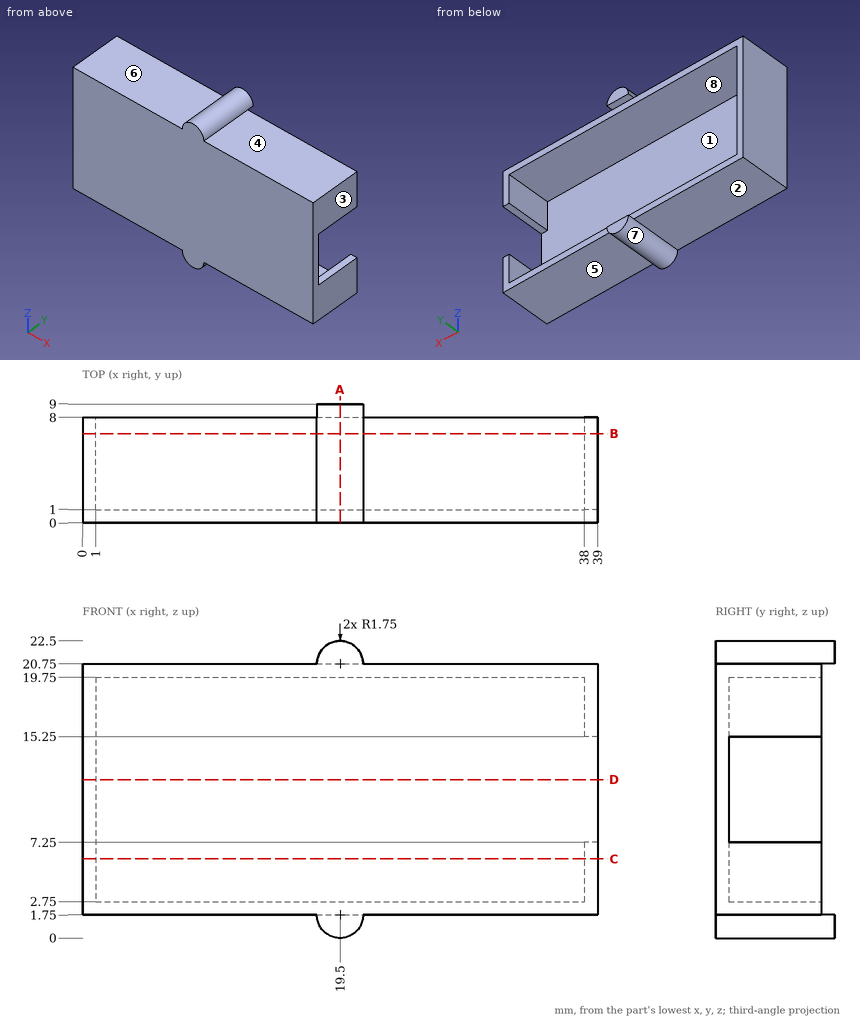
Check sheet for the drawn part. Datum: minimum x, y, z corner. Units: mm. A direction names the side the tool comes from. Coordinates: 2 decimals unless noted, no trailing zeros. Loops run counter-clockwise (first coordinate to the right, second up) from the corner with the lowest first, then second, coordinate; pieces in that order, holes last. Notation, with made-up numbers: (-9, 50) -> (25, 50) arc R14 cw to (25, 61) -> close; hole circle Ø9 at (26, 12.5). An arc over 180 degrees is marked (long way). Write each question's results on one line, items separated by ' | '.
Item 1: Section check D-D, the plane z = 12. Enter the section's corners in (x, y), plus the area to 3 significant figures.
Found:
outline: (0, 0) -> (39, 0) -> (39, 1) -> (1, 1) -> (1, 8) -> (0, 8) -> close | area: 46.0 mm2
Item 2: Section check B-B, the plane y = 6.75. Enter the section's corners in (x, z).
Found:
outline: (0, 1.75) -> (17.75, 1.75) arc R1.75 ccw to (21.25, 1.75) -> (39, 1.75) -> (39, 7.25) -> (38, 7.25) -> (38, 2.75) -> (1, 2.75) -> (1, 19.75) -> (38, 19.75) -> (38, 15.25) -> (39, 15.25) -> (39, 20.75) -> (21.25, 20.75) arc R1.75 ccw to (17.75, 20.75) -> (0, 20.75) -> close
Item 3: Tool access check on the marked faces 4, 5, 6, 7 and 8. Record the directions out of +Z, -Z, +X, -X, +Y, -Y that give a thin tool (end or side, any length) a straight path to the whole face; none if there is none.
Found:
face 4: +Z, +X, +Y, -Y | face 5: -Z, +X, +Y, -Y | face 6: +Z, -X, +Y, -Y | face 7: -Z, +Y, -Y | face 8: +Y
Item 4: Gauge pin test, flat ends, axial feed: pin 1 (4 mm diameter, centred on x = 30, y = 5, fed in from +Z); pin 2 (1.5 mm diameter, centred on x = 14, y = 3, fed in from -Z); pin 3 (8.5 mm diameter, centred on x = 25, z = 10, fed in from +Y). Record the tip position at first contact, or that the pin passes through.
Found:
pin 1: stops at z = 20.75 | pin 2: stops at z = 1.75 | pin 3: stops at y = 1
Item 5: Section check C-C, the plane z = 6. Enter the section's corners in (x, y), plus the area to 3 significant figures.
Found:
outline: (0, 0) -> (39, 0) -> (39, 8) -> (38, 8) -> (38, 1) -> (1, 1) -> (1, 8) -> (0, 8) -> close | area: 53.0 mm2
Item 6: Mould release check, pull along X, two halves, no side actions. Record for the marked faces 1, 2 and 3: +X half, -X half, draft (parallel to the pull), parting line (faces both ways), or undercut.
Found:
face 1: undercut | face 2: draft | face 3: +X half
Item 7: Material ranges on L1, parallel to Z at x = 32, y = 7; L2, parallel to X at y = 5, z = 4.75; L3, parallel to X at y = 4, z = 8.5, recorded low to high.
Found:
L1: z = 1.75 to 2.75, 19.75 to 20.75 | L2: x = 0 to 1, 38 to 39 | L3: x = 0 to 1
Item 8: Section check A-A, the plane x = 19.5. Enter the section's corners in (y, z), plus the area to 3 significant figures.
Found:
outline: (0, 0) -> (9, 0) -> (9, 1.75) -> (8, 1.75) -> (8, 2.75) -> (1, 2.75) -> (1, 19.75) -> (8, 19.75) -> (8, 20.75) -> (9, 20.75) -> (9, 22.5) -> (0, 22.5) -> close | area: 64.5 mm2
